from build123d import *

# Parameters (mm, degrees)
SKETCH2_R           = 32.5
BOSS_EXTRUDE1_DEPTH = 10
BOSS_EXTRUDE2_DEPTH = 2
CIRPATTERN1_COUNT   = 7
SKETCH4_R           = 12
BOSS_EXTRUDE3_DEPTH = 6
SKETCH5_R           = 10.5
BOSS_EXTRUDE4_DEPTH = 12
BOSS_EXTRUDE5_START = 8
SKETCH7_R           = 32.5
BOSS_EXTRUDE5_DEPTH = 8
SKETCH6_R           = 2
CUT_EXTRUDE1_DEPTH  = 50.360915713


with BuildPart() as part:
    # Sketch2 → Boss-Extrude1 (new body)
    with BuildSketch(Plane.XY):
        Circle(SKETCH2_R)
    extrude(amount=BOSS_EXTRUDE1_DEPTH)

    # Sketch3 → Boss-Extrude2 (add)
    with BuildSketch(Plane(origin=(0, 0, 0), x_dir=(0, 0, -1), z_dir=(1, 0, 0))):
        Polygon((-10, 32.5), (-19.587933614, 32.5), (-15, 28), (-15, 30), (-10, 30), align=None)
    boss_extrude2 = extrude(amount=BOSS_EXTRUDE2_DEPTH)

    # CirPattern1: Boss-Extrude2 ×7 about axis
    cirpattern1_axis = Axis((0, 0, 0), (0, 0, 1))
    for i in range(1, CIRPATTERN1_COUNT):
        add(boss_extrude2.rotate(cirpattern1_axis, i * 360 / CIRPATTERN1_COUNT))

    # Sketch4 → Boss-Extrude3 (add)
    with BuildSketch(Plane.XY.offset(10)):
        Circle(SKETCH4_R)
    extrude(amount=BOSS_EXTRUDE3_DEPTH)

    # Sketch5 → Boss-Extrude4 (add)
    with BuildSketch(Plane.XY.offset(10)):
        Circle(SKETCH5_R)
    extrude(amount=BOSS_EXTRUDE4_DEPTH)

    # Sketch7 → Boss-Extrude5 (add)
    with BuildSketch(Plane(origin=(0, 0, 0), x_dir=(-1, 0, 0), z_dir=(0, 0, -1)).offset(BOSS_EXTRUDE5_START)):
        Circle(SKETCH7_R)
    extrude(amount=-BOSS_EXTRUDE5_DEPTH)

    # Sketch6 → Cut-Extrude1 (cut, through all)
    with BuildSketch(Plane.XY.offset(10)):
        with Locations((23.5, 0)):
            Circle(SKETCH6_R)
        with Locations((11.75, -20.351596989)):
            Circle(SKETCH6_R)
        with Locations((-11.75, -20.351596989)):
            Circle(SKETCH6_R)
        with Locations((-23.5, 0)):
            Circle(SKETCH6_R)
        with Locations((-11.75, 20.351596989)):
            Circle(SKETCH6_R)
        with Locations((11.75, 20.351596989)):
            Circle(SKETCH6_R)
    extrude(amount=-CUT_EXTRUDE1_DEPTH, mode=Mode.SUBTRACT)


solid = part.part
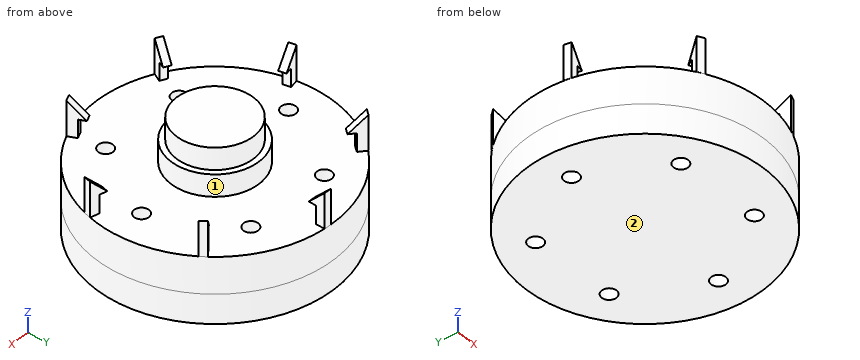
The listing builds one solid part. Answer for the finished solid, in the listing's coordinates (mm). Face numbers are marked on the shaded views. A direction names the side the tool comes from. Coordinates: 2 decimals unless noted, no trailing zeros. Loops run counter-clockwise (first coordinate to the right, second up) from the corner with the lowest first, then second, coordinate; pieces in that order, holes last. Notation, with made-up numbers: (45, -8.5) -> (104, -8.5) arc R25 cw to (104, 18.5) -> close; hole circle Ø6 at (61, -31.5). An arc over 180 degrees is marked (long way). Answer in a Markdown table with one row per item. Add a question column.
1. Flat-ended cylindrical pins translate along their axes: P1, Ø4, axis at x = -18.5, z = 11.5, coming from the -Y side; P2, Ø3, axis at x = 11.75, y = 20.35, coming from the +Z side; P3, Ø1.5, axis at y = -24.5, z = 4, coming from the -X side; P4, Ø8, axis at y = 9, z = 2, coming from the +X side. Find the tip coordinate at first contact, or state that the pin passes through.
2. The part is cut by section C-C, the plane y = 8. Write down the section's boundary in (x, z), then the cut area to 3 significant figures.
3. The part is cut by section A-A, the plane y = 0. Write down the section's boundary in (x, z).
4. The part is cut by section D-D, the plane y = 25.5. Write down the section's boundary in (x, z).
5. The part is cut by section B-B, the plane z = 8.75. Write down the section's boundary in (x, y).
6. Consider line 1 (X direction, y = 1, z = -4.75); line 2 (X direction, y = -20, z = 5); line 3 (Y direction, x = -11.75, z = -0.5). Determine where each line is inside the solid, lowest interval first. Write a range as [from, to].
7. For the marked faces 1 and 2, determine the directions among +Z, -Z, +X, -X, +Y, -Y from which every point of the face is accessible in a straight line to the end or side of a thin tool.
Answer below:
| question | item | result |
|---|---|---|
| 1 | P1 | y = -27.59 |
| 1 | P2 | through |
| 1 | P3 | x = -22.19 |
| 1 | P4 | x = 32.11 |
| 2 | outline | (-31.5, -8) -> (31.5, -8) -> (31.5, 10) -> (8.94, 10) -> (8.94, 16) -> (6.8, 16) -> (6.8, 22) -> (-6.8, 22) -> (-6.8, 16) -> (-8.94, 16) -> (-8.94, 10) -> (-31.5, 10) -> close |
| 2 | area | 1,320 mm2 |
| 3 | outline | (-32.5, -8) -> (-25.5, -8) -> (-25.5, 10) -> (-32.5, 10) -> close; (-21.5, -8) -> (21.5, -8) -> (21.5, 10) -> (12, 10) -> (12, 16) -> (10.5, 16) -> (10.5, 22) -> (-10.5, 22) -> (-10.5, 16) -> (-12, 16) -> (-12, 10) -> (-21.5, 10) -> close; (25.5, -8) -> (32.5, -8) -> (32.5, 10) -> (25.5, 10) -> close |
| 4 | outline | (-20.15, -8) -> (20.15, -8) -> (20.15, 10) -> (-20.15, 10) -> close |
| 5 | outline | circle Ø65 at (0, 0); hole circle Ø4 at (-23.5, 0); hole circle Ø4 at (-11.75, -20.35); hole circle Ø4 at (-11.75, 20.35); hole circle Ø4 at (11.75, -20.35); hole circle Ø4 at (11.75, 20.35); hole circle Ø4 at (23.5, 0) |
| 6 | line 1 | [-32.48, -25.23], [-21.77, 21.77], [25.23, 32.48] |
| 6 | line 2 | [-25.62, -13.72], [-9.78, 9.78], [13.72, 25.62] |
| 6 | line 3 | [-30.3, -22.35], [-18.35, 18.35], [22.35, 30.3] |
| 7 | face 1 | +Z |
| 7 | face 2 | -Z, +X, -X, +Y, -Y |
